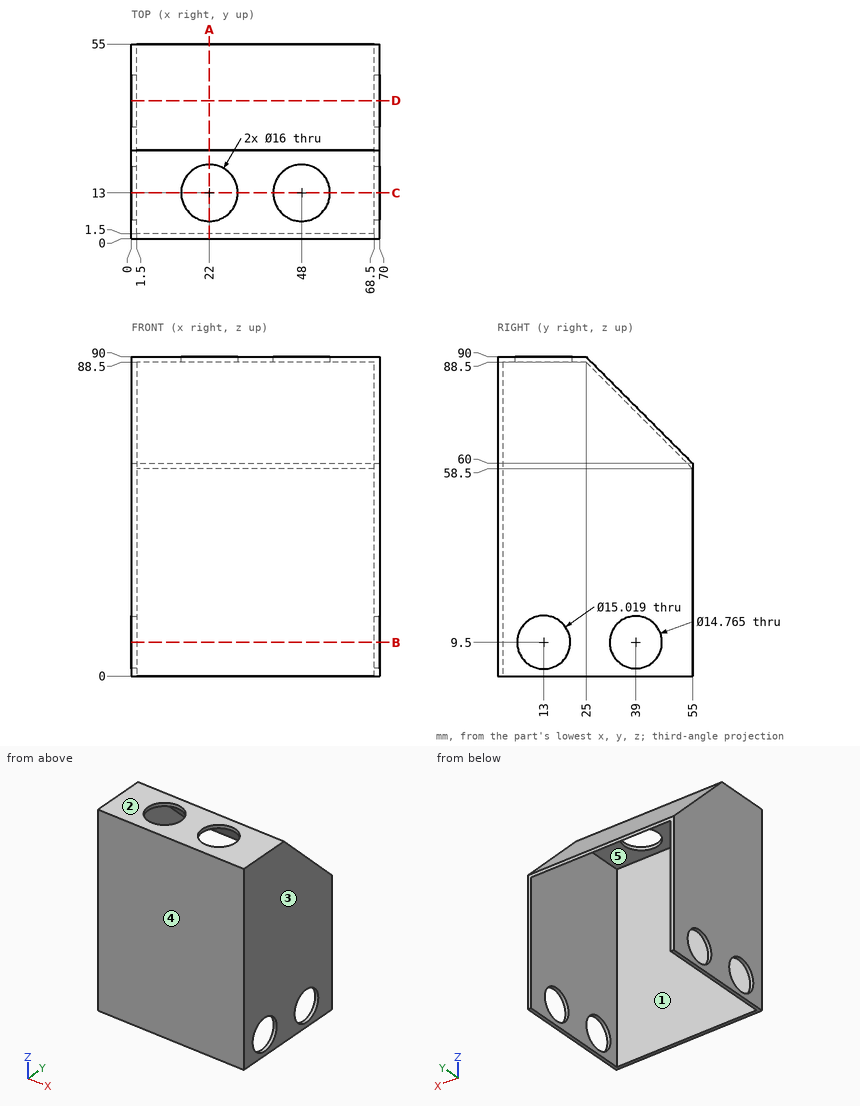
Drawing for the job (mm, zero at the part's lowest x, y, z). A direction names the side the tool comes from. Coordinates: 2 decimals unless noted, no trailing zeros. Order: outer loops, then holes, each group sorted by start corner. A loop starts at its lowest first (then second) coordinate and runs counter-clockwise, first axis right, second up.
Item 1: Drill centre lines: L1, parallel to Y at x = 1, z = 9; L2, parallel to X at y = 30.5, z = 80.5; L3, parallel to Y at x = 13.5, z = 40.5. Where is each one in solid material? Low to high.
Check sheet entries:
L1: y = 0 to 5.51, 20.49 to 31.63, 46.37 to 55
L2: x = 0 to 1.5, 68.5 to 70
L3: y = 0 to 1.5
Item 2: Band-saw the part on B-B on z = 9.5. List the corners of the cut face in (x, y), plus the area to 3 significant figures.
Check sheet entries:
outline: (0, 0) - (70, 0) - (70, 5.49) - (68.5, 5.49) - (68.5, 1.5) - (1.5, 1.5) - (1.5, 5.49) - (0, 5.49) - close; (0, 20.51) - (1.5, 20.51) - (1.5, 31.62) - (0, 31.62) - close; (0, 46.38) - (1.5, 46.38) - (1.5, 55) - (0, 55) - close; (68.5, 20.51) - (70, 20.51) - (70, 31.62) - (68.5, 31.62) - close; (68.5, 46.38) - (70, 46.38) - (70, 55) - (68.5, 55) - close
area: 176 mm2
Item 3: Band-saw the part on A-A on x = 22. List the corners of the cut face in (y, z).
Check sheet entries:
outline: (0, 0) - (1.5, 0) - (1.5, 88.5) - (5, 88.5) - (5, 90) - (0, 90) - close; (21, 88.5) - (25, 88.5) - (55, 58.5) - (55, 60) - (25, 90) - (21, 90) - close
Item 4: Band-saw the part on D-D on y = 39. List the corners of the cut face in (x, z), plus the area to 3 significant figures.
Check sheet entries:
outline: (0, 0) - (1.5, 0) - (1.5, 2.12) - (0, 2.12) - close; (0, 16.88) - (1.5, 16.88) - (1.5, 74.5) - (68.5, 74.5) - (68.5, 16.88) - (70, 16.88) - (70, 76) - (0, 76) - close; (68.5, 0) - (70, 0) - (70, 2.12) - (68.5, 2.12) - close
area: 284 mm2
Item 5: Band-saw the part on C-C on y = 13. List the corners of the cut face in (x, z).
Check sheet entries:
outline: (0, 0) - (1.5, 0) - (1.5, 1.99) - (0, 1.99) - close; (0, 17.01) - (1.5, 17.01) - (1.5, 88.5) - (14, 88.5) - (14, 90) - (0, 90) - close; (30, 88.5) - (40, 88.5) - (40, 90) - (30, 90) - close; (56, 88.5) - (68.5, 88.5) - (68.5, 17.01) - (70, 17.01) - (70, 90) - (56, 90) - close; (68.5, 0) - (70, 0) - (70, 1.99) - (68.5, 1.99) - close
Item 6: 3-axis set-ups, long thin cutter, end or side, ignore diameter. For the marked faces 1 and 2: which of +Z, -Z, +X, -X, +Y, -Y reach the whole face in a straight line?
Check sheet entries:
face 1: -Z
face 2: +Z, +X, -X, +Y, -Y
Item 7: Pin check, flat tips, straight feed: pin 1 Ø13.5 at (y, z) = (13, 9.5) entering from +X; pin 2 Ø21 at (x, y) = (22, 13) entering from -Z; pin 3 Ø23.5 at (y, z) = (39, 9.5) entering from +X; pin 4 Ø4 at (x, z) = (19.5, 43) entering from +Y. Stop position of each tip, or through.
Check sheet entries:
pin 1: passes through
pin 2: stops at z = 88.5
pin 3: stops at x = 70
pin 4: stops at y = 1.5
Item 8: Two-plate mould, pull along Y, no slides. Class the marked faces 3, 4 and 5: +Y half, -Y half, draft (parallel to the pull), parting line (faces both ways), or undercut.
Check sheet entries:
face 3: draft
face 4: -Y half
face 5: undercut
